The listing builds one solid part. Answer for the finished solid, in the listing's coordinates (mm). A direction names the side the tool comes from. Give positions to 0.01 mm unless a question says otherwise; leave off trailing zeros. Write each loop counter-clockwise with the first axis right and the second up, starting at its lowest first coordinate (ties: lowest second). Pieces come first, ordered by that corner, then holes. Notation, with made-up numbers: M 9,25.25 L 32,25.25 A32 ccw 32,59.25 Z; hole C -27,-5 d6. An arc over 180 degrees is marked long. Answer as a JSON object with one key per item and string values.
```python
from build123d import *

# Parameters (mm, degrees)
REVOLVE1_ANGLE = 180


with BuildPart() as part:
    # Sketch1 → Revolve1 (revolve)
    with BuildSketch(Plane.XY):
        with BuildLine():
            Line((-215, 0), (-215, 100))
            ThreePointArc((-215, 100), (-210.606601718, 110.606601718), (-200, 115))
            Line((-200, 115), (200, 115))
            ThreePointArc((200, 115), (210.606601718, 110.606601718), (215, 100))
            Line((215, 100), (215, 45))
            Line((215, 45), (285, 45))
            Line((285, 45), (285, 35))
            Line((285, 35), (200, 35))
            Line((200, 35), (200, 92.5))
            ThreePointArc((200, 92.5), (197.803300859, 97.803300859), (192.5, 100))
            Line((192.5, 100), (-192.5, 100))
            ThreePointArc((-192.5, 100), (-197.803300859, 97.803300859), (-200, 92.5))
            Line((-200, 92.5), (-200, 0))
            Line((-200, 0), (-215, 0))
        make_face()
    revolve(axis=Axis((0, 0, 0), (1, 0, 0)), revolution_arc=REVOLVE1_ANGLE)


solid = part.part
```
1. Consider line 1 along X through (y, z) = (42, 6.5); line 2 along X through (y, z) = (18, 86.5); line 3 along Y through (x, z) = (58.5, 86). Determine where each line is inside the solid, lowest interval first.
Verdict:
{"line 1": "x = -215 to -200, 200 to 285", "line 2": "x = -215 to -200, 200 to 215", "line 3": "y = -76.35 to -51.03, 51.03 to 76.35"}
2. A cutting plane is placed at C-C, the plane x = -147. Give the vertices of the cut face in (y, z).
Verdict:
{"outline": "M -115,0 L -100,0 A100 cw 100,0 L 115,0 A115 ccw Z"}
3. The mould has two halves that part along Y. Classify faces 5 (the flat face through (285, 3, 36)), 6 (the cylindrical face through (-2.695, 2.199, 99.976)), 7 (the cylindrical face through (2.8, 2.529, 114.972)): released by +Y, released by -Y, zero draft, split by the parting line, or undercut.
Verdict:
{"face 5": "zero draft", "face 6": "undercut", "face 7": "split by the parting line"}
4. For faces 1 (the flat face through (-1, -102, 0)), 2 (the flat face through (-200, -1, 37)), 3 (the cylindrical face through (241.9, 0.77, 34.99)), 4 (the flat face through (215, -1, 51)), determine the directions among +Z, -Z, +X, -X, +Y, -Y from which every point of the face is accessible in a straight line to the end or side of a thin tool.
Verdict:
{"face 1": "-Z, +X, -X, +Y, -Y", "face 2": "-Z", "face 3": "-Z, +X", "face 4": "+Z, +X"}
5. A cutting plane is placed at B-B, the plane x = 228. Give the vertices of the cut face in (y, z).
Verdict:
{"outline": "M -45,0 L -35,0 A35 cw 35,0 L 45,0 A45 ccw Z"}
6. Flat-ended cylindrical pins translate along their axes: pin 1 (12 mm diameter, centred on y = -78, z = 99.5, fed in from -X); pin 2 (6 mm diameter, centred on x = -107.5, y = 60.5, fed in from -Z); pin 3 (3 mm diameter, centred on x = 151.5, y = 83, fed in from +Z); pin 4 (8 mm diameter, centred on x = 197.5, z = 32, fed in from +Y). Find the tip coordinate at first contact, or state that the pin passes through.
Verdict:
{"pin 1": "passes through", "pin 2": "stops at z = 77.25", "pin 3": "stops at z = 81.13", "pin 4": "stops at y = 111.54"}
7. A cutting plane is placed at A-A, the plane y = 0. Give the vertices of the cut face in (x, z), plus the area to 3 significant figures.
Verdict:
{"outline": "M -215,0 L -200,0 L -200,92.5 A7.5 cw -192.5,100 L 192.5,100 A7.5 cw 200,92.5 L 200,35 L 285,35 L 285,45 L 215,45 L 215,100 A15 ccw 200,115 L -200,115 A15 ccw -215,100 Z", "area": "9,550 mm2"}
